Build history of the part. All positions in model axes, mm. Face numbers are marked on the shaded views. A direction names the side the tool comes from. Coordinates: 2 decimals unless noted, no trailing zeros. Order: outer loops, then holes, each group sorted by start corner. A loop starts at its lowest first (then second) coordinate and runs counter-clockwise, first axis right, second up. Notation, with made-up numbers: (44.25, 67) - (57.25, 67) arc R31 ccw to (57.25, 102) - close; hole circle Ø4 at (74, 7). An arc over 180 degrees is marked (long way). Write each question's results on one line, items separated by ' | '.
from build123d import *

# Parameters (mm, degrees)
PAD010_DEPTH    = 9
ARRAY001_COUNT  = 8
SKETCH014_R     = 5.2
SKETCH014_R_2   = 4.25
PAD009_DEPTH    = 9
SKETCH017_R     = 4.5
POCKET005_DEPTH = 2
CHAMFER004_SIZE = 0.2


with BuildPart() as array001:
    # Sketch015 → Pad010 (new body)
    with BuildSketch(Plane.XY):
        with BuildLine():
            Line((1, 6.0174745533), (1, 4.7674745533))
            Line((1, 4.7674745533), (-1, 4.7674745533))
            Line((-1, 4.7674745533), (-1, 6.0174745533))
            ThreePointArc((1, 6.0174745533), (0, 6.1), (-1, 6.0174745533))
        make_face()
    extrude(amount=PAD010_DEPTH)


with BuildPart() as array001_1:
    # Body005 placement: moved
    add(array001.part.moved(Location((0, 0, -3))))

    # Array001: Array001 ×8 about axis
    array001_axis = Axis((0, 0, 0), (0, 0, 1))


with BuildPart() as array001_2:
    add(array001_1.part)
    for i in range(1, ARRAY001_COUNT):
        add(array001_1.part.rotate(array001_axis, i * 360 / ARRAY001_COUNT))


with BuildPart() as chamfer004:
    # Sketch014 → Pad009 (new body)
    with BuildSketch(Plane.XY):
        Circle(SKETCH014_R)
        Circle(SKETCH014_R_2, mode=Mode.SUBTRACT)
    extrude(amount=PAD009_DEPTH)

    # Sketch017 (on Face3 of Pad009) → Pocket005 (cut)
    with BuildSketch(Plane(origin=(0, 0, 0), x_dir=(1, 0, 0), z_dir=(0, 0, -1))):
        Circle(SKETCH017_R)
    extrude(amount=-POCKET005_DEPTH, mode=Mode.SUBTRACT)


with BuildPart() as chamfer004_1:
    # Body004 placement: moved
    add(chamfer004.part.moved(Location((0, 0, -3))))

    # Fusion: union Array001
    add(array001_2.part)

    # Chamfer004
    chamfer004_edges = [chamfer004_1.edges().sort_by_distance(p)[0] for p in [
        (1.989954, 4.804174, -3),
        (1.989954, 4.804174, 6),
        (1, 5.560207, -3),
        (1, 5.560207, 6),
        (1, 6.017475, 1.5),
        (3.224554, 4.638767, -3),
        (3.54789, 4.962104, 1.5),
        (3.224554, 4.638767, 6),
        (-1, 6.017475, 1.5),
        (0, 6.1, -3),
        (0, 6.1, 6),
        (-1.989954, 4.804174, -3),
        (-1.989954, 4.804174, 6),
        (-3.224554, 4.638767, -3),
        (-3.224554, 4.638767, 6),
        (-3.54789, 4.962104, 1.5),
        (-1, 5.560207, -3),
        (-1, 5.560207, 6),
        (-4.962104, 3.54789, 1.5),
        (-4.313351, 4.313351, -3),
        (-4.313351, 4.313351, 6),
        (-4.804174, 1.989954, -3),
        (-4.804174, 1.989954, 6),
        (-5.560207, 1, -3),
        (-5.560207, 1, 6),
        (-6.017475, 1, 1.5),
        (-4.638767, 3.224554, -3),
        (-4.638767, 3.224554, 6),
        (-6.017475, -1, 1.5),
        (-6.1, 0, -3),
        (-6.1, 0, 6),
        (-4.804174, -1.989954, 6),
        (-4.804174, -1.989954, -3),
        (-4.638767, -3.224554, -3),
        (-4.638767, -3.224554, 6),
        (-4.962104, -3.54789, 1.5),
        (-5.560207, -1, -3),
        (-5.560207, -1, 6),
        (-3.54789, -4.962104, 1.5),
        (-4.313351, -4.313351, -3),
        (-4.313351, -4.313351, 6),
        (-1.989954, -4.804174, 6),
        (-1.989954, -4.804174, -3),
        (-1, -5.560207, -3),
        (-1, -5.560207, 6),
        (-1, -6.017475, 1.5),
        (-3.224554, -4.638767, -3),
        (-3.224554, -4.638767, 6),
        (1, -6.017475, 1.5),
        (0, -6.1, -3),
        (0, -6.1, 6),
        (1.989954, -4.804174, 6),
        (1.989954, -4.804174, -3),
        (3.224554, -4.638767, -3),
        (3.224554, -4.638767, 6),
        (3.54789, -4.962104, 1.5),
        (1, -5.560207, -3),
        (1, -5.560207, 6),
        (4.962104, -3.54789, 1.5),
        (4.313351, -4.313351, -3),
        (4.313351, -4.313351, 6),
        (5.560207, -1, -3),
        (5.560207, -1, 6),
        (6.017475, -1, 1.5),
        (6.017475, 1, 1.5),
        (6.1, 0, -3),
        (6.1, 0, 6),
        (5.560207, 1, -3),
        (5.560207, 1, 6),
        (4.804174, -1.989954, 6),
        (4.804174, -1.989954, -3),
        (4.804174, 1.989954, -3),
        (4.804174, 1.989954, 6),
        (4.638767, -3.224554, -3),
        (4.638767, -3.224554, 6),
        (4.638767, 3.224554, -3),
        (4.638767, 3.224554, 6),
        (4.962104, 3.54789, 1.5),
        (4.313351, 4.313351, -3),
        (4.313351, 4.313351, 6),
        (-4.5, 0, -3),
        (-4.25, 0, -1),
        (-4.25, 0, 6),
    ]]
    chamfer(chamfer004_edges, length=CHAMFER004_SIZE)


with BuildPart() as chamfer004_2:
    # Chamfer004 placement: moved
    add(chamfer004_1.part.moved(Location((0, 0, 0.5))))


solid = chamfer004_2.part
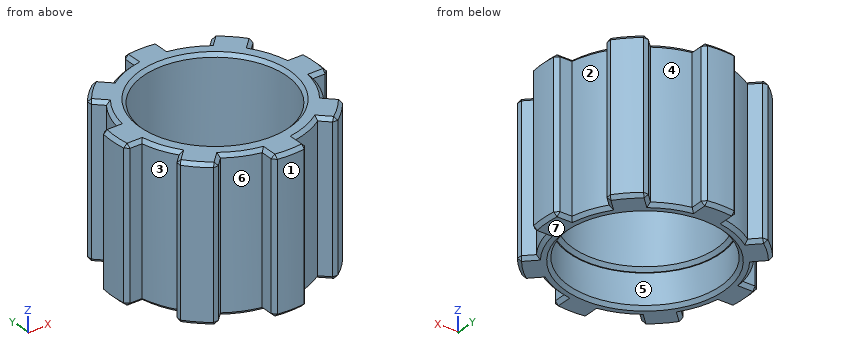
1. Band-saw the part on A-A on x = 0. Give the cut face in (y, z), then the cut area to 3 significant figures.
Solved:
outline: (-6.1, -2.3) - (-5.9, -2.5) - (-4.7, -2.5) - (-4.5, -2.3) - (-4.5, -0.5) - (-4.45, -0.5) - (-4.25, -0.3) - (-4.25, 6.3) - (-4.45, 6.5) - (-5.9, 6.5) - (-6.1, 6.3) - close; (4.25, -0.3) - (4.45, -0.5) - (4.5, -0.5) - (4.5, -2.3) - (4.7, -2.5) - (5.9, -2.5) - (6.1, -2.3) - (6.1, 6.3) - (5.9, 6.5) - (4.45, 6.5) - (4.25, 6.3) - close | area: 32.1 mm2
2. Two-plate mould, pull along Y, no slides. Class the marked faces 1, 2, 3 and 4: +Y half, -Y half, draft (parallel to the pull), parting line (faces both ways), or undercut.
Solved:
face 1: -Y half | face 2: undercut | face 3: undercut | face 4: +Y half
3. Band-saw the part on C-C on y = -5.5. Give the cut face in (x, z).
Solved:
outline: (-1, -2.3) - (-0.8, -2.5) - (0.8, -2.5) - (1, -2.3) - (1, 6.3) - (0.8, 6.5) - (-0.8, 6.5) - (-1, 6.3) - close
4. Tool access for the marked faces 5, 6 and 7: list every direction of +Z, -Z, +X, -X, +Y, -Y with a clear straight run to the whole face (end or side of a thin tool).
Solved:
face 5: -Z | face 6: +Z, -Z, -Y | face 7: -Z, +X, -X, +Y, -Y
5. Probe line 1 (Y direction, x = 0, z = 2.5); line 2 (X direction, y = 4.75, z = 4); line 3 (X direction, y = 0, z = -1.6). List the from-to ranges inside material, lowest first.
Solved:
line 1: y = -6.1 to -4.25, 4.25 to 6.1 | line 2: x = -3.83 to -3.34, -2.12 to 2.12, 3.34 to 3.83 | line 3: x = -6.1 to -4.5, 4.5 to 6.1
6. Drop flat-ended pins along their axis: pin 1 Ø0.6 at (x, z) = (5.5, 1) entering from +Y; pin 2 Ø6 at (x, y) = (-5, 3.5) entering from +Z; pin 3 Ø0.6 at (x, z) = (-5.5, 0) entering from -Y; pin 4 Ø3 at (y, z) = (4, -1.5) entering from +X. Give the stop position or say it passes through.
Solved:
pin 1: stops at y = 1 | pin 2: stops at z = 6.5 | pin 3: stops at y = -1 | pin 4: stops at x = 4.84
